Autodesk Inventor part; units mm, degrees
ref_plane "YZ Plane" through (0, 0, 0) normal (1, 0, 0) x (0, 1, 0)
ref_plane "XZ Plane" through (0, 0, 0) normal (0, 1, 0) x (-1, 0, 0)
ref_plane "XY Plane" through (0, 0, 0) normal (0, 0, 1) x (1, 0, 0)
sketch "スケッチ1" plane through (0, 0, 0) normal (0, 0, 1) x (1, 0, 0)
  circle A0 centre (0, 27) radius 16 construction
  circle A1 centre (0, 46) radius 1
  line L0 (0, 60.4716) -> (0, -64.9114) construction
  circle A2 centre (0, 27) radius 15 construction
  line L1 (1.5, 47.5) -> (-1.5, 47.5)
  line L2 (-1.5, 47.5) -> (-1.5, 44.5)
  line L3 (-1.5, 44.5) -> (1.5, 44.5)
  line L4 (1.5, 44.5) -> (1.5, 47.5)
  line L5 (1.5, 44.5) -> (1.5, 42.9295)
  line L6 (-1.5, 44.5) -> (-1.5, 42.9295)
  circle A3 centre (21.5, 19) radius 1.5 construction
  circle A4 centre (-21.5, 19) radius 1.5 construction
  line L7 (0, 27) -> (21.5, 19) construction
  line L8 (0, 27) -> (-21.5, 19) construction
  circle A5 centre (0, 27) radius 10
  circle A6 centre (0, 27) radius 5
  line L9 (-1.5, 44.5) -> (-1.5, 36.8869)
  line L10 (1.5, 44.5) -> (1.5, 36.8869)
  line L11 (-22.0231, 20.4058) -> (-9.7893, 24.958) construction
  line L12 (-20.9769, 17.5942) -> (-8.7431, 22.1463) construction
  line L13 (22.0231, 20.4058) -> (9.7893, 24.958) construction
  line L14 (20.9769, 17.5942) -> (8.7431, 22.1463) construction
  circle A7 centre (0, 27) radius 1
  circle A8 centre (21.5, 19) radius 1.05
  circle A9 centre (-21.5, 19) radius 1.05
  line L15 (19.5, 21) -> (23.5, 21) construction
  line L16 (23.5, 21) -> (23.5, 17) construction
  line L17 (23.5, 17) -> (19.5, 17) construction
  line L18 (19.5, 17) -> (19.5, 21) construction
  line L19 (19.5, 21) -> (23.5, 17) construction
  line L20 (23.5, 21) -> (19.5, 17) construction
  line L21 (9.7893, 24.958) -> (20.4263, 21)
  line L22 (20.4263, 21) -> (23.5, 21)
  line L23 (23.5, 21) -> (23.5, 17)
  line L24 (23.5, 17) -> (19.5, 17)
  line L25 (19.5, 17) -> (19.5, 18.1437)
  line L26 (19.5, 18.1437) -> (8.7431, 22.1463)
  line L27 (-23.5, 17) -> (-19.5, 17) construction
  line L28 (-19.5, 17) -> (-19.5, 21) construction
  line L29 (-19.5, 21) -> (-23.5, 21) construction
  line L30 (-23.5, 21) -> (-23.5, 17) construction
  line L31 (-23.5, 17) -> (-19.5, 21) construction
  line L32 (-19.5, 17) -> (-23.5, 21) construction
  line L33 (-9.7893, 24.958) -> (-20.4263, 21)
  line L34 (-20.4263, 21) -> (-23.5, 21)
  line L35 (-23.5, 21) -> (-23.5, 17)
  line L36 (-23.5, 17) -> (-19.5, 17)
  line L37 (-19.5, 17) -> (-19.5, 18.1437)
  line L38 (-19.5, 18.1437) -> (-8.7431, 22.1463)
  line L39 (-40.2847, 27) -> (38.7153, 27) construction
  point P0 (0, 0)
  dimension "d0" = 32
  dimension "d1" = 2
  dimension "d3" = 27
  dimension "d4" = 30
  dimension "d5" = 3
  dimension "d6" = 3
  dimension "d8" = 1.5
  dimension "d15" = 20
  dimension "d16" = 10
  dimension "d20" = 2
  dimension "d29" = 27
  dimension "d30" = 27
  dimension "d32" = 3
  dimension "d33" = 3
  dimension "d35" = 2.1
  dimension "d36" = 2.1
  dimension "d40" = 4
  dimension "d41" = 4
  dimension "d42" = 4
  dimension "d43" = 4
  dimension "d48" = 19
  dimension "d49" = 1.5
  dimension "d50" = 21.5
  dimension "d51" = 21.5
extrude "押し出し1" add sketch "スケッチ1" against normal blind 16 contours A1 | L4 L3 L2 L1
extrude "押し出し3" cut sketch "スケッチ1" against normal blind 4 contours A1
sketch "スケッチ6" plane through (0, 0, 0) normal (0, 0, 1) x (1, 0, 0)
  circle A0 centre (0, 27) radius 5
  circle A1 centre (0, 27) radius 5
  point P0 (0, 0)
  dimension "d23" = 10
sketch "スケッチ7" plane through (0, 0, -16) normal (0, 0, -1) x (-1, 0, 0)
  circle A0 centre (0, 46) radius 1
  point P0 (0, 0)
extrude "押し出し7" cut sketch "スケッチ7" against normal blind 3.5
extrude "押し出し9" add sketch "スケッチ1" against normal blind 4 contours L5 L10 A5 L9 L6 L3 | A5 | A5 L38 L37 L36 L35 L34 L33 | L21 L22 L23 L24 L25 L26 A5 | A6
extrude "押し出し10" cut sketch "スケッチ6" against normal blind 3.5
sketch "スケッチ8" plane through (0, 0, 0) normal (0, 0, 1) x (1, 0, 0)
  circle A0 centre (0, 27) radius 5
  circle A1 centre (21.5, 19) radius 1.05
  circle A2 centre (-21.5, 19) radius 1.05
  circle A3 centre (0, 46) radius 1
  line L0 (1.5, 47.5) -> (-1.5, 47.5)
  line L1 (-1.5, 47.5) -> (-1.5, 36.8869)
  arc A4 (-1.5, 36.8869) -> (-9.7893, 24.958) centre (0, 27) ccw
  line L2 (-9.7893, 24.958) -> (-20.4263, 21)
  line L3 (-20.4263, 21) -> (-23.5, 21)
  line L4 (-23.5, 21) -> (-23.5, 17)
  line L5 (-23.5, 17) -> (-19.5, 17)
  line L6 (-19.5, 17) -> (-19.5, 18.1437)
  line L7 (-19.5, 18.1437) -> (-8.7431, 22.1463)
  arc A5 (-8.7431, 22.1463) -> (8.7431, 22.1463) centre (0, 27) ccw
  line L8 (8.7431, 22.1463) -> (19.5, 18.1437)
  line L9 (19.5, 18.1437) -> (19.5, 17)
  line L10 (19.5, 17) -> (23.5, 17)
  line L11 (23.5, 17) -> (23.5, 21)
  line L12 (23.5, 21) -> (20.4263, 21)
  line L13 (20.4263, 21) -> (9.7893, 24.958)
  arc A6 (9.7893, 24.958) -> (1.5, 36.8869) centre (0, 27) ccw
  line L14 (1.5, 36.8869) -> (1.5, 47.5)
  circle A7 centre (0, 27) radius 1
  point P0 (0, 0)
equation "\"d30\" = d29"
equation "\"d33\" = d32"
equation "\"d36\" = d35"
equation "\"d41\" = d40"
equation "\"d42\" = d40"
equation "\"d43\" = d40"
equation "\"d51\" = d50"
properties part number "s_mount"
Check sheet for the modelled part. Datum: model origin and axes. Units: mm. A direction names the side the tool comes from. Give positions to 0.01 mm unless a question says otherwise; leave off trailing zeros. Loops run counter-clockwise (first coordinate to the right, second up) from the corner with the lowest first, then second, coordinate; pieces in that order, holes last. Notation, with made-up numbers: M -18.75,6.25 L -10.75,6.25 A25 cw -10.75,35.25 Z; hole C 10,-36.5 d7. An arc over 180 degrees is marked long. Answer as a JSON object with one key per item and string values. Group by question number.
Q1. Cross-section at B-B on y = 27. Record the cut outline in (x, z).
Q2. Cross-section at D-D on z = -14.5. Record the cut outline in (x, y).
Q3. Access from +Z, -Z, +X, -X, +Y, -Y to the whole of each face (thin tool, end or side, straight path). Record for faces 4 (the flat face through (-14.197, 20.117, -1.972)), 5 (the flat face through (1.5, 46, -4)), 6 (the cylindrical face through (-1.08, 22.12, -1.73)), 7 (the cylindrical face through (0, 47, -14)), 8 (the flat face through (-1.5, 45, -6)).
Q4. Cross-section at A-A on x = 0. Record the cut outline in (y, z).
Q5. Cross-section at C-C on y = 46. Record the cut outline in (x, z), then the cut area to 3 significant figures.
Q6. Go/stop test with flat-tipped pins: P1, Ø3, axis at y = 34, z = -2, coming from the +X side; P2, Ø5, axis at x = -1.5, y = 26.5, coming from the +Z side; P3, Ø3, axis at x = 0, y = 27, coming from the -Z side. Record where each tip stops, or that it passes through.
Q7. Release check for a two-part mould opening along X. For faces 1 (the cylindrical face through (8, 33, -2)), 2 (the flat face through (22, 21, -2)), 3 (the flat face through (0, 46, -4)) record: released by +X, released by -X, zero draft, split by the parting line, or undercut.
Q8. Material ranges on line 1 along Y through (x, z) = (21.5, -1.4); line 2 along Z through (x, y) = (4, 23.5); line 3 along Y through (x, z) = (21, -3), recorded low to high. Write a range as [from, to].
Evaluation:
{
 "1": {"outline": "M -10,-4 L -1,-4 L -1,-3.5 L -5,-3.5 L -5,0 L -10,0 Z; M 1,-4 L 10,-4 L 10,0 L 5,0 L 5,-3.5 L 1,-3.5 Z"},
 "2": {"outline": "M -1.5,44.5 L 1.5,44.5 L 1.5,47.5 L -1.5,47.5 Z; hole C 0,46 d2"},
 "3": {"face 4": "+Z, -Z, -Y", "face 5": "+Z, -Z, +X, +Y", "face 6": "+Z", "face 7": "-Z", "face 8": "+Z, -Z, -X, +Y"},
 "4": {"outline": "M 17,-4 L 26,-4 L 26,-3.5 L 22,-3.5 L 22,0 L 17,0 Z; M 28,-4 L 44.5,-4 L 44.5,-16 L 45,-16 L 45,-12.5 L 47,-12.5 L 47,-16 L 47.5,-16 L 47.5,0 L 47,0 L 47,-4 L 45,-4 L 45,0 L 32,0 L 32,-3.5 L 28,-3.5 Z"},
 "5": {"outline": "M -1.5,-16 L -1,-16 L -1,-12.5 L 1,-12.5 L 1,-16 L 1.5,-16 L 1.5,0 L 1,0 L 1,-4 L -1,-4 L -1,0 L -1.5,0 Z", "area": "33.0 mm2"},
 "6": {"P1": "stops at x = 8.35", "P2": "stops at z = -3.5", "P3": "stops at z = -4"},
 "7": {"face 1": "released by +X", "face 2": "zero draft", "face 3": "undercut"},
 "8": {"line 1": "y = [17, 17.95], [20.05, 21]", "line 2": "z = [-4, 0]", "line 3": "y = [17, 18.08], [19.92, 21]"}
}
